Input: dimensioned drawing with shaded views. Units: mm. Origin: part minimum x, y, z. Round coordinates to 2 decimals unless told otherwise and drop trailing zeros. Write each loop counter-clockwise with the first axis right and the second up, starting at its lowest first coordinate (ties: lowest second). Pieces come first, ordered by that corner, then holes. Notation, with made-up numbers: M -9,69 L 47,69 A29 cw 47,92 Z; hole C 8,20 d9. An arc over 180 degrees is marked long. Use one line per item in the form item = value. Start each with the question number.
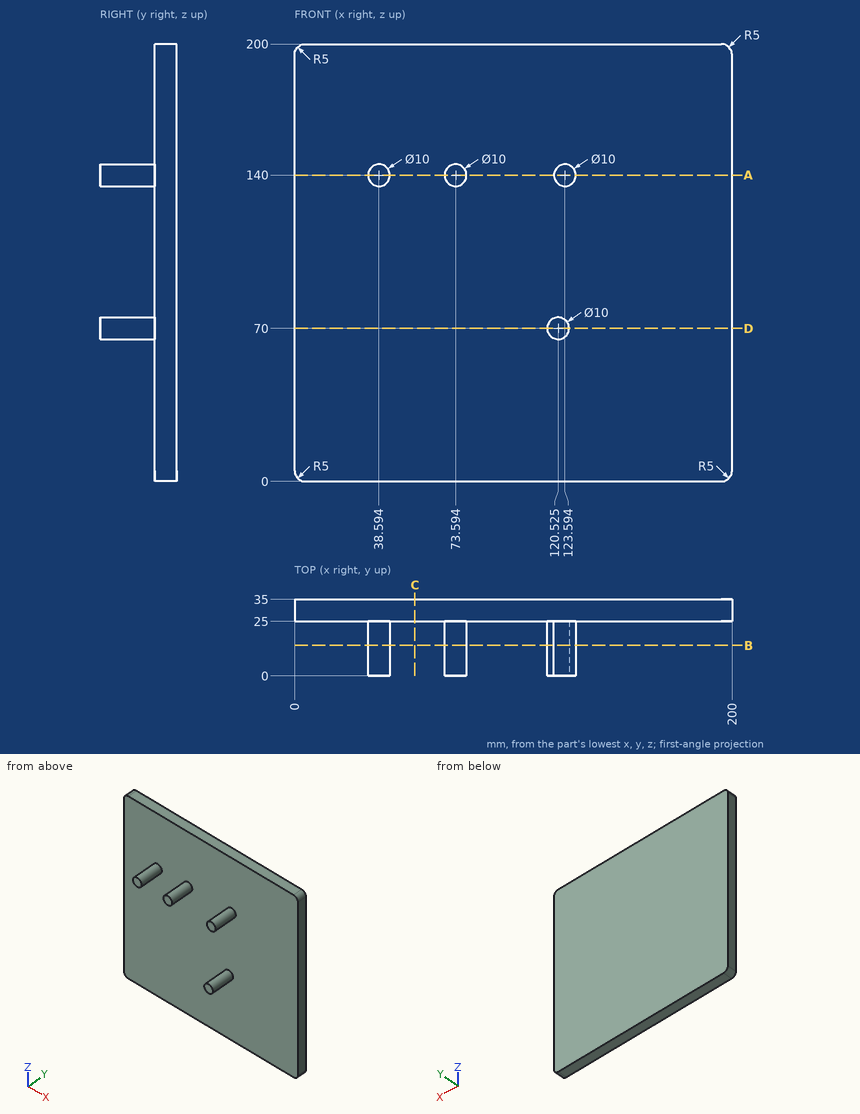
1. Section query C-C (x = 55). Return loops of the section in (y, z), then the cut area to 3 significant figures.
2. Ray query, probe 1 along X at (y, z) = (8, 136); probe 2 along Y at (x, z) = (89, 45.5); probe 3 along X at (y, z) = (2, 71.5) (1 decimal). Return the intervals inside material, ascending.
3. Section query D-D (z = 70). Return loops of the section in (x, y) (3 decimals), then the cut area to 3 significant figures.
4. Contact query for flat-ended pins moving along their axis: pin 1 (1 mm diameter, centred on x = 73, y = 7.5, fed in from +Z); pin 2 (4 mm diameter, centred on x = 78, y = 17.5, fed in from -Z); pin 3 (6 mm diameter, centred on y = 6, z = 75.5, fed in from +X) (3 decimals). Output: stop coordinate, or through.
5. Section query A-A (z = 140). Return loops of the section in (x, y).
6. Section query B-B (y = 14). Return loops of the section in (x, z) (3 decimals).
Checks:
q1.outline = M 25,0 L 35,0 L 35,200 L 25,200 Z
q1.area = 2,000 mm^2
q2.probe_1 = 35.59 to 41.59, 70.59 to 76.59, 120.59 to 126.59
q2.probe_2 = 25 to 35
q2.probe_3 = 115.8 to 125.3
q3.outline = M 0,25 L 115.525,25 L 115.525,0 L 125.525,0 L 125.525,25 L 200,25 L 200,35 L 0,35 Z
q3.area = 2,250 mm^2
q4.pin_1 = 145
q4.pin_2 = 135.62
q4.pin_3 = 124.855
q5.outline = M 0,25 L 33.59,25 L 33.59,0 L 43.59,0 L 43.59,25 L 68.59,25 L 68.59,0 L 78.59,0 L 78.59,25 L 118.59,25 L 118.59,0 L 128.59,0 L 128.59,25 L 200,25 L 200,35 L 0,35 Z
q6.outline = C 38.594,140 d10; C 73.594,140 d10; C 120.525,70 d10; C 123.594,140 d10
